Geometry check sheet. Reference: the model listing, model coordinates, mm. Face numbers are marked on the shaded views. A direction names the side the tool comes from. Coordinates: 2 decimals unless noted, no trailing zeros. Write each loop counter-clockwise with the first axis right and the second up, starting at its lowest first coordinate (ties: lowest second). Pieces come first, ordered by that corner, then holes. Notation, with made-up numbers: (57, -9.75) -> (102, -9.75) arc R29 ccw to (102, 11.25) -> close; hole circle Ø4 at (32.25, 7). An arc over 180 degrees is marked (long way). One line per question, with ' | ' between items.
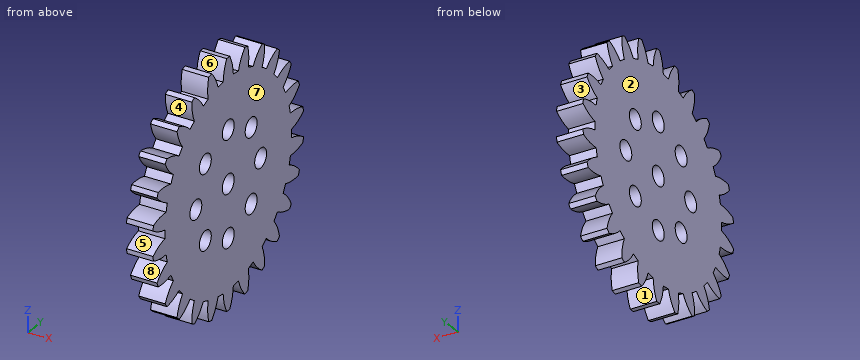
from build123d import *

# Parameters (mm, degrees)
BASPROSKE_W         = 3
BASPROSKE_H         = 14
TOOTHCUT_DEPTH      = 21.024984395
TEETHCUTS_COUNT     = 26
TEETHCUTS_ANGLE     = 346.153846154
BORSKE_R            = 4
BORE_DEPTH          = 50.0000508
EXTRUDE_START       = -3
SKETCH_1_R          = 4
EXTRUDE_1_DEPTH     = 3
SKETCH_2_R          = 1.1
CUT_EXTRUDE_1_DEPTH = 3


with BuildPart() as part:
    # BasProSke → Base-Revolve (revolve)
    with BuildSketch(Plane(origin=(0, 0, 0), x_dir=(1, 0, 0), z_dir=(0, 1, 0)), mode=Mode.PRIVATE) as base_revolve_sk:
        with Locations((1.5, 7)):
            Rectangle(BASPROSKE_W, BASPROSKE_H)
    revolve(base_revolve_sk.sketch.rotate(Axis((-10, 0, 0), (1, 0, 0)), 180), axis=Axis((-10, 0, 0), (1, 0, 0)))

    # TooCutSke → ToothCut (cut, through all)
    with BuildSketch(Plane(origin=(0, 0, 0), x_dir=(0, 0, -1), z_dir=(1, 0, 0))):
        with BuildLine():
            ThreePointArc((0.476965065, 11.739314517), (0, 11.749), (-0.476965065, 11.739314517))
            ThreePointArc((-0.476965065, 11.739314517), (-0.82065865, 12.901686978), (-1.424117301, 13.952911348))
            ThreePointArc((-1.424117301, 13.952911348), (0, 14.0254), (1.424117301, 13.952911348))
            ThreePointArc((1.424117301, 13.952911348), (0.82065865, 12.901686978), (0.476965065, 11.739314517))
        make_face()
    toothcut = extrude(amount=TOOTHCUT_DEPTH, mode=Mode.SUBTRACT)

    # TeethCuts: ToothCut ×26 about axis
    teethcuts_axis = Axis((-10, 0, 0), (1, 0, 0))
    for i in range(1, TEETHCUTS_COUNT):
        add(toothcut.rotate(teethcuts_axis, i * TEETHCUTS_ANGLE / (TEETHCUTS_COUNT - 1)), mode=Mode.SUBTRACT)

    # BorSke → Bore (cut, symmetric)
    with BuildSketch(Plane(origin=(0, 0, 0), x_dir=(0, 0, -1), z_dir=(1, 0, 0))):
        with Locations(Location((0, 0, 0), (0, 0, 180))):
            Circle(BORSKE_R)
    extrude(amount=BORE_DEPTH, both=True, mode=Mode.SUBTRACT)

    # ｽｹｯﾁ1 → ﾎﾞｽ - 押し出し1 (add)
    with BuildSketch(Plane.ZY.offset(EXTRUDE_START)):
        Circle(SKETCH_1_R)
    extrude(amount=EXTRUDE_1_DEPTH)

    # ｽｹｯﾁ2 → ｶｯﾄ - 押し出し1 (cut)
    with BuildSketch(Plane.ZY):
        Circle(SKETCH_2_R)
        with Locations((0, 6)):
            Circle(SKETCH_2_R)
        with Locations((4.242640687, 4.242640687)):
            Circle(SKETCH_2_R)
        with Locations((6, 0)):
            Circle(SKETCH_2_R)
        with Locations((4.242640687, -4.242640687)):
            Circle(SKETCH_2_R)
        with Locations((0, -6)):
            Circle(SKETCH_2_R)
        with Locations((-4.242640687, -4.242640687)):
            Circle(SKETCH_2_R)
        with Locations((-6, 0)):
            Circle(SKETCH_2_R)
        with Locations((-4.242640687, 4.242640687)):
            Circle(SKETCH_2_R)
    extrude(amount=-CUT_EXTRUDE_1_DEPTH, mode=Mode.SUBTRACT)


solid = part.part
1. Cross-section at A-A on z = 6.25. Record the boundary of the cut face in (x, y).
Worked answers:
outline: (0, -10.61) -> (3, -10.61) -> (3, -1.07) -> (0, -1.07) -> close; (0, 1.07) -> (3, 1.07) -> (3, 10.61) -> (0, 10.61) -> close
2. Mould release check, pull along Z, two halves, no side actions. Record for the marked faces 6, 7 and 8: released by +Z, released by -Z, zero draft, split by the parting line, or undercut.
Worked answers:
face 6: released by +Z | face 7: zero draft | face 8: undercut
3. Material ranges on line 1 (Z direction, x = 0.3, y = 12); line 2 (Z direction, x = 0.2, y = 4.25); line 3 (Y direction, x = 2.6, z = -10.5), recorded low to high. Write a range as from..to.
Worked answers:
line 1: -5.28..-3.65, -2.36..-0.53, 0.53..2.36, 3.65..5.28 | line 2: -10.95..-5.34, -3.14..3.14, 5.34..10.95 | line 3: -9.26..-8.66, -6.5..6.5, 8.66..9.26
4. Go/stop test with flat-tipped pins: P1, Ø1.8, axis at y = 4.24, z = -4.24, coming from the -X side; P2, Ø1, axis at x = 1.5, z = 4, coming from the -Y side. Record where each tip stops, or that it passes through.
Worked answers:
P1: through | P2: y = -13.01
5. Cross-section at B-B on x = 0.35. Give the number of separate pieces and of enclosed holes in the cut face, and give its area (3 significant figures).
Worked answers:
separate pieces: 1 | enclosed holes: 9 | area: 482 mm²
6. Tool access check on the marked faces 1, 2, 3, 4 and 5. Record the directions out of +Z, -Z, +X, -X, +Y, -Y that give a thin tool (end or side, any length) a straight path to the whole face; none if there is none.
Worked answers:
face 1: -Z, +X, -X | face 2: +Z, -Z, -X, +Y, -Y | face 3: +X, -X, +Y | face 4: +X, -X | face 5: +X, -X, -Y
